The model under review builds one solid part; all positions refer to its coordinate system, in mm. A direction names the side the tool comes from. Give positions to 0.01 mm unless a question says otherwise; leave off trailing zeros. Order: outer loops, then holes, each group sorted by start corner. A loop starts at its lowest first (then second) coordinate and runs counter-clockwise, first axis right, second up. Notation, with made-up numbers: (-4.75, 59) -> (5.25, 59) arc R13 cw to (5.25, 84) -> close; hole circle Ø8 at (-10, -1.5). An arc over 180 degrees is marked (long way). Use one line per item in the form item = value.
```python
from build123d import *

# Parameters (mm, degrees)
SKETCH2_W                = 10
SKETCH2_H                = 5
BOSS_EXTRUDE1_DEPTH      = 10
SKETCH3_R                = 2
BOSS_EXTRUDE2_DEPTH      = 3.333333333
BOSS_EXTRUDE3_START      = -3.333333333
SKETCH4_R                = 2
BOSS_EXTRUDE3_DEPTH      = 3.333333333
BOSS_EXTRUDE4_DEPTH      = 1.5
BOSS_EXTRUDE4_DEPTH_BACK = 1.5
SKETCH6_R                = 2
BOSS_EXTRUDE5_DEPTH      = 1.5
BOSS_EXTRUDE5_DEPTH_BACK = 1.5
CUT_EXTRUDE1_DEPTH       = 18.501785659


with BuildPart() as part:
    # Sketch2 → Boss-Extrude1 (new body)
    with BuildSketch(Plane(origin=(0, 0, 0), x_dir=(0, 0, -1), z_dir=(1, 0, 0))):
        with Locations((5, 2.5)):
            Rectangle(SKETCH2_W, SKETCH2_H)
    extrude(amount=BOSS_EXTRUDE1_DEPTH)

    # Sketch3 → Boss-Extrude2 (add)
    with BuildSketch(Plane.ZY):
        with BuildLine():
            Line((2.5, 5), (0, 5))
            Line((0, 5), (0, 2.5))
            ThreePointArc((0, 2.5), (4.267766953, 0.732233047), (2.5, 5))
        make_face()
        with Locations((2.5, 2.5)):
            Circle(SKETCH3_R, mode=Mode.SUBTRACT)
    extrude(amount=-BOSS_EXTRUDE2_DEPTH)

    # Sketch4 → Boss-Extrude3 (add)
    with BuildSketch(Plane(origin=(10, 0, 0), x_dir=(0, 0, -1), z_dir=(1, 0, 0)).offset(BOSS_EXTRUDE3_START)):
        with BuildLine():
            Line((-2.5, 5), (0, 5))
            Line((0, 5), (0, 2.5))
            ThreePointArc((0, 2.5), (-4.267766953, 0.732233047), (-2.5, 5))
        make_face()
        with Locations(Location((-2.5, 2.5, 0), (0, 0, 180))):
            Circle(SKETCH4_R, mode=Mode.SUBTRACT)
    extrude(amount=BOSS_EXTRUDE3_DEPTH)

    # Sketch6 → Boss-Extrude4 (add, two sides: drawn at the far end of the back side and taken through both)
    with BuildSketch(Plane.ZY.offset(-5).offset(-BOSS_EXTRUDE4_DEPTH_BACK)):
        with BuildLine():
            Line((-12.5, 5), (-10, 5))
            Line((-10, 5), (-10, 2.5))
            ThreePointArc((-10, 2.5), (-14.267766953, 0.732233047), (-12.5, 5))
        make_face()
        with Locations((-12.5, 2.5)):
            Circle(SKETCH6_R, mode=Mode.SUBTRACT)
    extrude(amount=BOSS_EXTRUDE4_DEPTH + BOSS_EXTRUDE4_DEPTH_BACK)

    # Sketch8 → Boss-Extrude5 (add, two sides: drawn at the far end of the back side and taken through both)
    with BuildSketch(Plane.ZY.offset(-5).offset(-BOSS_EXTRUDE5_DEPTH_BACK)):
        with BuildLine():
            Line((0, 5), (-2, 5))
            Line((-2, 5), (-5.2, 5))
            Line((-5.2, 5), (-5.2, 5.04))
            add(Edge.make_bspline(
                [(-2, 6.25), (-2.494910157, 6.25), (-3.057241258, 5.810278687), (-3.866517232, 5.241546577), (-4.160995323, 5.04), (-5.2, 5.04)],
                knots=[0, 0, 0, 0, 0.415212535, 0.515212535, 1, 1, 1, 1], degree=3))
            Line((-2, 6.25), (8, 6.25))
            Line((8, 6.25), (8, 5))
            Line((8, 5), (0, 5))
        make_face()
    extrude(amount=BOSS_EXTRUDE5_DEPTH + BOSS_EXTRUDE5_DEPTH_BACK)

    # Sketch9 → Cut-Extrude1 (cut, through all)
    with BuildSketch(Plane.ZY.offset(-3.5)):
        Polygon((8, 6.25), (5.805296546, 6.25), (5.805296546, 5.167226788), (2.5, 5.167226788), (2.5, 5), (8, 5), align=None)
    extrude(amount=-CUT_EXTRUDE1_DEPTH, mode=Mode.SUBTRACT)


solid = part.part
```
1. Add section A-A on y = 1.25. Give the boundary of the cut face in (x, z).
Values:
outline = (0, -10) -> (10, -10) -> (10, 0) -> (0, 0) -> close; (0, 0.33) -> (3.33, 0.33) -> (3.33, 0.94) -> (0, 0.94) -> close; (0, 4.06) -> (3.33, 4.06) -> (3.33, 4.67) -> (0, 4.67) -> close; (3.5, -14.67) -> (6.5, -14.67) -> (6.5, -14.06) -> (3.5, -14.06) -> close; (3.5, -10.94) -> (6.5, -10.94) -> (6.5, -10.33) -> (3.5, -10.33) -> close; (6.67, 0.33) -> (10, 0.33) -> (10, 0.94) -> (6.67, 0.94) -> close; (6.67, 4.06) -> (10, 4.06) -> (10, 4.67) -> (6.67, 4.67) -> close
2. For pin 1 Ø3 at (x, z) = (5.5, -3) entering from +Y; pin 2 Ø2 at (x, y) = (3.5, 2.5) entering from +Z; pin 3 Ø6 at (x, z) = (7.5, -6.5) entering from +Y; pin 4 Ø5 at (x, z) = (7, -11.5) entering from +Y, all flat-tipped, find the tip position at first contact; note any pin that passes through.
Values:
pin_1 = 6.25
pin_2 = 5
pin_3 = 5.38
pin_4 = 5
3. Add section B-B on z = -11.75. Give the boundary of the cut face in (x, y), then the cut area to 3 significant figures.
Values:
outline = (3.5, 0.12) -> (6.5, 0.12) -> (6.5, 0.65) -> (3.5, 0.65) -> close; (3.5, 4.35) -> (6.5, 4.35) -> (6.5, 5) -> (3.5, 5) -> close
area = 3.53 mm^2
4. For L1, parallel to Y at x = 0.75, z = 2.5; L2, parallel to X at y = 4.25, z = 1; L3, parallel to X at y = 5.5, z = -0.25, list the stretches that pass through material, from the lowest coordinate up.
Values:
L1 = 0 to 0.5, 4.5 to 5
L2 = 0 to 3.33, 6.67 to 10
L3 = 3.5 to 6.5
5. The part is to be moulded in two halves that separate along Y. For faces 6 (the face through (5, 1.3, -14.1)), 7 (the face through (5, 0, -5)), 8 (the face through (6.667, 4, 0.8)), say which applies: +Y half, -Y half, draft (parallel to the pull), parting line (faces both ways), or undercut.
Values:
face_6 = undercut
face_7 = -Y half
face_8 = draft
6. Add section D-D on y = 3.25. Give the boundary of the cut face in (x, z).
Values:
outline = (0, -10) -> (3.5, -10) -> (3.5, -10.65) -> (6.5, -10.65) -> (6.5, -10) -> (10, -10) -> (10, 0.65) -> (6.67, 0.65) -> (6.67, 0) -> (3.33, 0) -> (3.33, 0.65) -> (0, 0.65) -> close; (0, 4.35) -> (3.33, 4.35) -> (3.33, 4.88) -> (0, 4.88) -> close; (3.5, -14.88) -> (6.5, -14.88) -> (6.5, -14.35) -> (3.5, -14.35) -> close; (6.67, 4.35) -> (10, 4.35) -> (10, 4.88) -> (6.67, 4.88) -> close
7. Add section C-C on z = -0.5. Give the boundary of the cut face in (x, y), then the cut area to 4 significant figures.
Values:
outline = (0, 0) -> (10, 0) -> (10, 5) -> (6.5, 5) -> (6.5, 6.25) -> (3.5, 6.25) -> (3.5, 5) -> (0, 5) -> close
area = 53.75 mm^2
8. Tool access review of faces 1 (the face through (6.5, 6, 2)), 2 (the face through (5, 5.167, 4)), 3 (the face through (3.333, 4, 0.8)), 4 (the face through (5, 5, 1)), 5 (the face through (6.5, 4, -10.8)): name each direction out of +Z, -Z, +X, -X, +Y, -Y from which nothing blocks a thin tool from reaching the whole face with its end or side.
Values:
face_1 = +Z, -Z, +X, +Y
face_2 = +Z, +X, -X, -Y
face_3 = +Z, +Y, -Y
face_4 = +Z, -Y
face_5 = -Z, +X, +Y, -Y
